Autodesk Inventor part; units mm, degrees
ref_plane "YZ Plane" through (0, 0, 0) normal (1, 0, 0) x (0, 1, 0)
ref_plane "XZ Plane" through (0, 0, 0) normal (0, 1, 0) x (-1, 0, 0)
ref_plane "XY Plane" through (0, 0, 0) normal (0, 0, 1) x (1, 0, 0)
sketch "Sketch1" plane through (0, 0, 0) normal (0, 0, 1) x (1, 0, 0)
  circle A0 centre (0, 0) radius 44.925
  circle A1 centre (0, 0) radius 57.417 construction
  circle A2 centre (-57.417, 0) radius 2.1
  circle A3 centre (0, -57.417) radius 2.1
  circle A4 centre (57.417, 0) radius 2.1
  circle A5 centre (0, 57.417) radius 2.1
  circle A6 centre (0, 0) radius 41.75
  line L0 (0, 62.3245) -> (4.25, 59.8707)
  line L1 (4.25, 59.8707) -> (4.25, 54.9633)
  line L2 (4.25, 54.9633) -> (0, 52.5095)
  line L3 (0, 52.5095) -> (-4.25, 54.9633)
  line L4 (-4.25, 54.9633) -> (-4.25, 59.8707)
  line L5 (-4.25, 59.8707) -> (0, 62.3245)
  line L6 (60.1041, 10.6066) -> (10.6066, 60.1041)
  line L7 (-10.6066, 60.1041) -> (-60.1041, 10.6066)
  line L8 (-60.1041, -10.6066) -> (-10.6066, -60.1041)
  line L9 (10.6066, -60.1041) -> (60.1041, -10.6066)
  arc A7 (-10.6066, -60.1041) -> (10.6066, -60.1041) centre (0, -49.4975) ccw
  arc A8 (-60.1041, 10.6066) -> (-60.1041, -10.6066) centre (-49.4975, 0) ccw
  arc A9 (10.6066, 60.1041) -> (-10.6066, 60.1041) centre (0, 49.4975) ccw
  arc A10 (60.1041, -10.6066) -> (60.1041, 10.6066) centre (49.4975, 0) ccw
  line L10 (-59.8707, -4.25) -> (-62.3245, 0)
  line L11 (-54.9633, -4.25) -> (-59.8707, -4.25)
  line L12 (-62.3245, 0) -> (-59.8707, 4.25)
  line L13 (-59.8707, 4.25) -> (-54.9633, 4.25)
  line L14 (-54.9633, 4.25) -> (-52.5095, 0)
  line L15 (-52.5095, 0) -> (-54.9633, -4.25)
  line L16 (4.25, -59.8707) -> (0, -62.3245)
  line L17 (4.25, -54.9633) -> (4.25, -59.8707)
  line L18 (0, -62.3245) -> (-4.25, -59.8707)
  line L19 (-4.25, -59.8707) -> (-4.25, -54.9633)
  line L20 (-4.25, -54.9633) -> (0, -52.5095)
  line L21 (0, -52.5095) -> (4.25, -54.9633)
  line L22 (59.8707, 4.25) -> (62.3245, 0)
  line L23 (54.9633, 4.25) -> (59.8707, 4.25)
  line L24 (62.3245, 0) -> (59.8707, -4.25)
  line L25 (59.8707, -4.25) -> (54.9633, -4.25)
  line L26 (54.9633, -4.25) -> (52.5095, 0)
  line L27 (52.5095, 0) -> (54.9633, 4.25)
  point P0 (70.7107, 0)
  point P1 (0, 70.7107)
  point P2 (-70.7107, 0)
  point P3 (0, -70.7107)
  dimension "d1" = 114.834
  dimension "d0" = 89.85
  dimension "d2" = 4.2
  dimension "d5" = 360
  dimension "d8" = 83.5
  dimension "d18" = 8.5
  dimension "d25" = 100
  dimension "d26" = 100
  dimension "d27" = 15
  dimension "d30" = 360
extrude "Extrusion1" add sketch "Sketch1" along normal blind 7 contours L0 L1 L2 L3 L4 L5 | A10 L9 A7 L8 A8 L7 A9 L6 | L10 L12 L13 L14 L15 L11 | L16 L18 L19 L20 L21 L17 | L22 L24 L25 L26 L27 L23
extrude "Extrusion2" add sketch "Sketch1" along normal blind 4 contours A0
extrude "Extrusion3" cut sketch "Sketch1" along normal blind 4 contours A2 | A3 | A4 | A5 | L0 L1 L2 L3 L4 L5 | L10 L12 L13 L14 L15 L11 | L16 L18 L19 L20 L21 L17 | L22 L24 L25 L26 L27 L23
properties part number "Fix_bearing_Base"
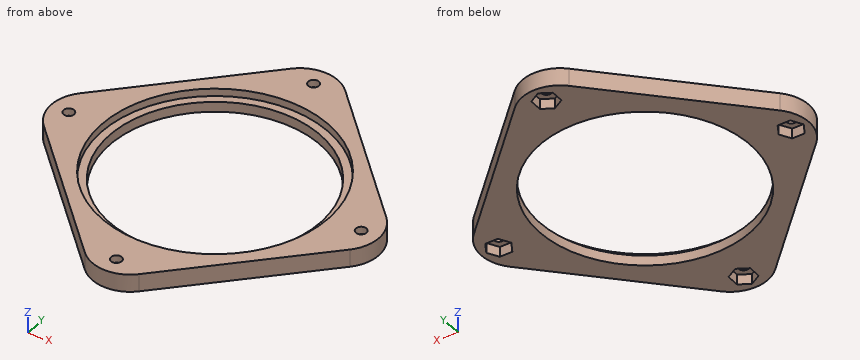
Here's how the part is built. I have some questions about the finished solid (model axes, mm). Coordinates: 2 decimals unless noted, no trailing zeros. Write each loop counter-clockwise with the first axis right and the second up, starting at its lowest first coordinate (ties: lowest second). Pieces come first, ordered by that corner, then holes. Notation, with made-up numbers: M 42,87.25 L 101,87.25 A12 ccw 101,97.25 Z; hole C 73,37.25 d3. An arc over 180 degrees is marked long. Answer as CSV lines item,"result". Start each with the question number.
Q1. Suppose I cut it at C-C, the plane y = 51. List the corners of the cut face in (x, z) for me, then the cut area to 3 significant figures.
Q2. Suppose I cut it at A-A, the plane z = 2. State how many separate pieces and enclosed holes the cut face has, then the cut area to 3 significant figures.
Q3. Suppose I cut it at B-B, the plane x = 35.5. List the corners of the cut face in (y, z) for me.
Q4. I need wall thicknesses on probe 1 along Y at (x, z) = (0, 5) (1 decimal); probe 2 along X at (y, z) = (-20, 6); probe 3 along X at (y, z) = (-17, 0.75). Which ranges of each line are inside material? Lowest first, please. Write a range as [from, to].
Q5. Will these pins go through, and if not, where does the flat tip stop? pin 1 Ø3 at (y, z) = (-58, 3) entering from -X; pin 2 Ø3 at (x, z) = (58, 1) entering from -Y; pin 3 Ø5 at (x, y) = (-57.417, 0) entering from -Z; pin 4 Ø2.5 at (x, y) = (0, -57.417) entering from +Z.
Entries:
1,outline,"M -19.71,0 L 19.71,0 L 19.71,7 L -19.71,7 Z"
1,area,"276 mm²"
2,separate pieces,"1"
2,enclosed holes,"5"
2,area,"4,080 mm²"
3,outline,"M -35.21,0 L -21.97,0 L -21.97,4 L -27.53,4 L -27.53,7 L -35.21,7 Z; M 21.97,0 L 35.21,0 L 35.21,7 L 27.53,7 L 27.53,4 L 21.97,4 Z"
4,probe 1,"y = [-64.5, -59.5], [-55.3, -44.9], [44.9, 55.3], [59.5, 64.5]"
4,probe 2,"x = [-50.71, -40.23], [40.23, 50.71]"
4,probe 3,"x = [-53.71, -38.13], [38.13, 53.71]"
5,pin 1,"stops at x = -14.21"
5,pin 2,"stops at y = -14.21"
5,pin 3,"stops at z = 4"
5,pin 4,"passes through"
